Autodesk Inventor part; units mm, degrees
ref_plane "YZ Plane" through (0, 0, 0) normal (1, 0, 0) x (0, 1, 0)
ref_plane "XZ Plane" through (0, 0, 0) normal (0, 1, 0) x (-1, 0, 0)
ref_plane "XY Plane" through (0, 0, 0) normal (0, 0, 1) x (1, 0, 0)
sketch "Esboço1" plane through (0, 0, 0) normal (0, 0, 1) x (1, 0, 0)
  circle A0 centre (0, 0) radius 8
  dimension "d0" = 16
extrude "Extrusão1" add sketch "Esboço1" along normal blind 651
sketch "Esboço2" plane through (0, 0, 651) normal (0, 0, 1) x (1, 0, 0)
  circle A0 centre (0, 0) radius 6
  dimension "d3" = 12
extrude "Extrusão2" add sketch "Esboço2" along normal blind 39
sketch "Esboço3" plane through (0, 0, 690) normal (0, 0, 1) x (1, 0, 0)
  circle A0 centre (0, 0) radius 5
  dimension "d6" = 10
extrude "Extrusão3" add sketch "Esboço3" along normal blind 15
sketch "Esboço4" plane through (0, 0, 0) normal (0, 0, -1) x (-1, 0, 0)
  circle A0 centre (0, 0) radius 5
  dimension "d9" = 10
extrude "Extrusão4" add sketch "Esboço4" along normal blind 9.15
sketch "Esboço5" plane through (0, 0, -9.15) normal (0, 0, -1) x (-1, 0, 0)
  circle A0 centre (0, 0) radius 4.5
  dimension "d12" = 9
extrude "Extrusão5" add sketch "Esboço5" along normal blind 1.15
sketch "Esboço6" plane through (0, 0, -10.3) normal (0, 0, -1) x (-1, 0, 0)
  circle A0 centre (0, 0) radius 5
  dimension "d15" = 10
extrude "Extrusão6" add sketch "Esboço6" along normal blind 1.85
thread "Rosca1"
chamfer "Chanfro1" distance 0.5 angle 45 5 edges at (-5, 0, 705) (-6, 0, 690) (-8, 0, 651) (-8, 0, 0) (5, 0, -12.15)
properties part number "SFU16XX_X"
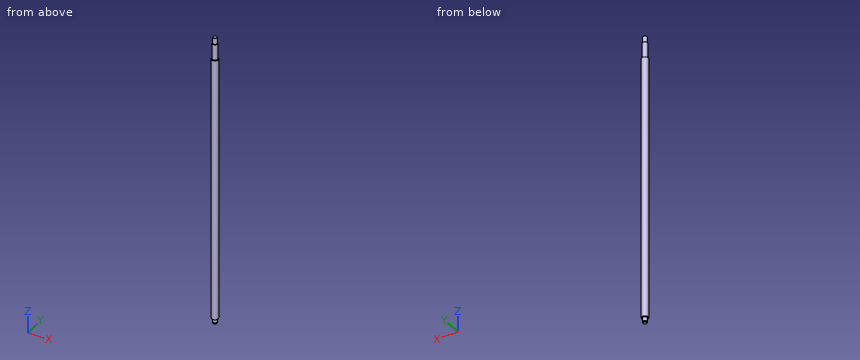
Work out the finished part from the listing and answer in its coordinate system (mm). Give positions to 0.01 mm unless a question says otherwise; leave off trailing zeros. Order: outer loops, then holes, each group sorted by start corner. A loop starts at its lowest first (then second) coordinate and runs counter-clockwise, first axis right, second up. Notation, with made-up numbers: M 39.25,48.25 L 86.25,48.25 A19 ccw 86.25,80.25 Z; hole C 77,55.5 d1. An arc over 180 degrees is marked long. Return JSON: item names as keys, results as strings.
Q1. Find section C-C, the plane z = 356. Write down the section's boundary in (x, y), and give its area (3 significant figures).
Answer below:
{"outline": "C 0,0 d16", "area": "201 mm^2"}
Q2. Find the intervals of material crossed by line 1 along Y through (x, z) = (5.25, 44.5); line 2 along Z through (x, y) = (6, -2.5); line 3 along X through (y, z) = (-6.25, 254), in increasing order. Write a range as [from, to].
Answer below:
{"line 1": "y = [-6.04, 6.04]", "line 2": "z = [0, 651]", "line 3": "x = [-4.99, 4.99]"}
Q3. Each of these flat-tipped pins is pushed along its axis until it touches: pin 1 (5 mm diameter, centred on y = -5, z = 321.5, fed in from +X); pin 2 (2 mm diameter, centred on y = 6, z = 587.5, fed in from +X) (3 decimals); pin 3 (3 mm diameter, centred on y = 2.5, z = 116, fed in from +X). Where does it stop, or does it pass through?
Answer below:
{"pin 1": "stops at x = 7.6", "pin 2": "stops at x = 6.245", "pin 3": "stops at x = 7.94"}
